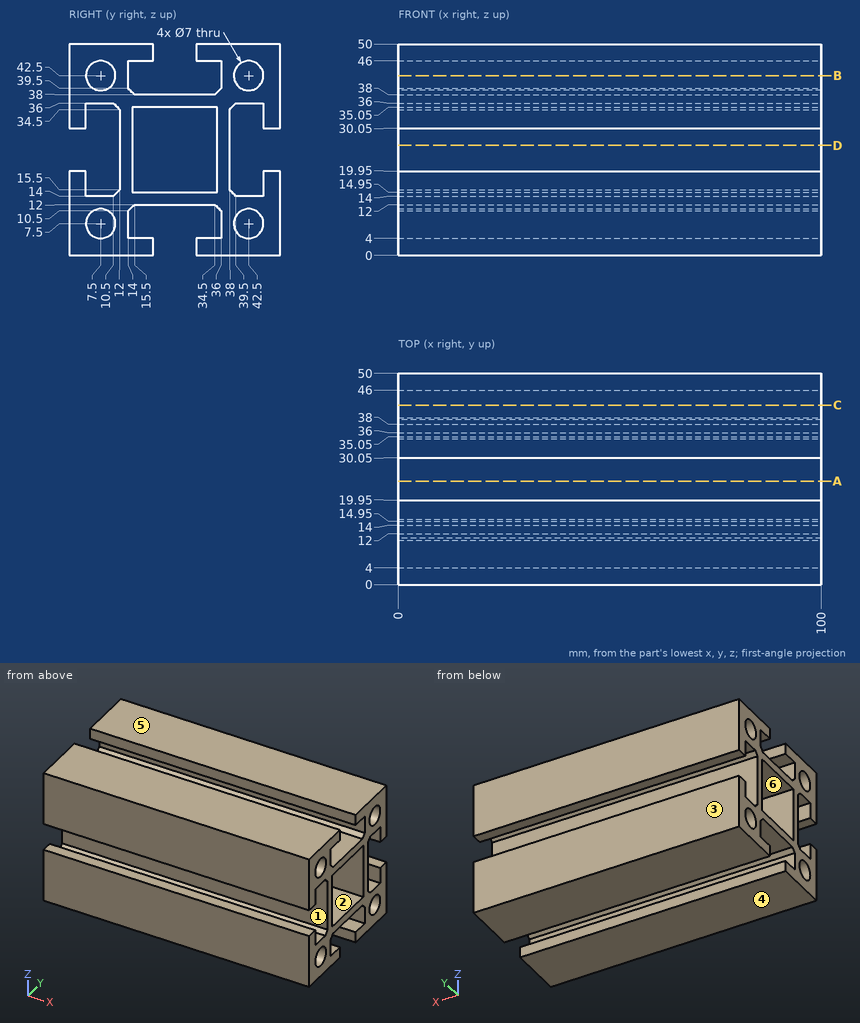
Could you check a few things on this drawing? It's one solid part, dimensions in mm from its lowest x, y, z. A direction names the side the tool comes from. Coordinates: 2 decimals unless noted, no trailing zeros. Write each loop counter-clockwise with the first axis right and the second up, starting at its lowest first coordinate (ties: lowest second). Pieces come first, ordered by that corner, then holes. Notation, with made-up numbers: (20.25, 68) - (77.25, 68) arc R30 cw to (77.25, 96) - close; hole circle Ø7 at (54, -1.5). An arc over 180 degrees is marked (long way). Put each result on its own line as item: value. Start each with the question number.
Q1. I'm going to push flat-ended pins straight in: P1, Ø6.5, axis at y = 42.5, z = 42.5, coming from the +X side; P2, Ø6, axis at x = 33.5, y = 25.5, coming from the +Z side. Where does each tip first touch, or does it pass through?
Q2. I want a section at A-A on y = 24.5. Write out the boundary of the cut face in (x, z).
Q3. Thinking about a two-plate mould opening in Y: for the marked faces 1, 2, 3 and 4, which applies, pulls with the +Y half, pulls with the -Y half, needs draft (parallel to the pull), parting line crosses it, or undercut?
Q4. Please list where these lines run through material, in increasing order: L1, parallel to Y at x = 75, z = 42.5; L2, parallel to Z at x = 30, y = 16.
Q5. I want a section at B-B on z = 42.5. Write out the boundary of the cut face in (x, y).
Q6. Which directions (+Z, -Z, +X, -X, +Y, -Y) give clear straight access to the entire face, cutting with the end or side of a thin tool? Please do the marked faces 5 and 6.
Checks:
1. P1: through
1. P2: z = 38
2. outline: (0, 12) - (100, 12) - (100, 14.95) - (0, 14.95) - close; (0, 35.05) - (100, 35.05) - (100, 38) - (0, 38) - close
3. face 1: undercut
3. face 2: undercut
3. face 3: pulls with the +Y half
3. face 4: needs draft
4. L1: 0 to 4, 11 to 14, 36 to 39, 46 to 50
4. L2: 0 to 4, 12 to 14.95, 35.05 to 38, 46 to 50
5. outline: (0, 0) - (100, 0) - (100, 4) - (0, 4) - close; (0, 11) - (100, 11) - (100, 14) - (0, 14) - close; (0, 36) - (100, 36) - (100, 39) - (0, 39) - close; (0, 46) - (100, 46) - (100, 50) - (0, 50) - close
6. face 5: +Z, +X, -X, +Y, -Y
6. face 6: +X, -X
